```python
from build123d import *

# Parameters (mm, degrees)
SKETCH1_R           = 37.5
BOSS_EXTRUDE1_DEPTH = 65
CHAMFER1_SIZE       = 25
CHAMFER1_SIZE2      = 12.738136237
SKETCH3_R           = 21
CUT_EXTRUDE1_DEPTH  = 30
SKETCH4_R           = 35
CUT_EXTRUDE2_DEPTH  = 39
SKETCH5_R           = 24.761863763
BOSS_EXTRUDE3_DEPTH = 30
SKETCH6_R           = 21
CUT_EXTRUDE3_DEPTH  = 28
SKETCH7_R           = 20
CUT_EXTRUDE4_DEPTH  = 30


with BuildPart() as part:
    # Sketch1 → Boss-Extrude1 (new body)
    with BuildSketch(Plane(origin=(0, 0, 0), x_dir=(1, 0, 0), z_dir=(0, 1, 0))):
        with Locations(Location((0, 0, 0), (0, 0, 270))):
            Circle(SKETCH1_R)
    extrude(amount=BOSS_EXTRUDE1_DEPTH)

    # Chamfer1
    chamfer1_edges = [part.edges().sort_by_distance(p)[0] for p in [
        (0, 65, -37.5),
    ]]
    chamfer1_side = [part.faces().sort_by_distance(p)[0] for p in [
        (0, 32.5, -37.5),
    ]]
    chamfer(chamfer1_edges, length=CHAMFER1_SIZE, length2=CHAMFER1_SIZE2, reference=chamfer1_side[0])

    # Sketch3 → Cut-Extrude1 (cut)
    with BuildSketch(Plane(origin=(0, 65, 0), x_dir=(1, 0, 0), z_dir=(0, 1, 0))):
        with Locations(Location((0, 0, 0), (0, 0, 270))):
            Circle(SKETCH3_R)
    extrude(amount=-CUT_EXTRUDE1_DEPTH, mode=Mode.SUBTRACT)

    # Sketch4 → Cut-Extrude2 (cut)
    with BuildSketch(Plane.XZ):
        with Locations(Location((0, 0, 0), (0, 0, 270))):
            Circle(SKETCH4_R)
    extrude(amount=-CUT_EXTRUDE2_DEPTH, mode=Mode.SUBTRACT)

    # Sketch5 → Boss-Extrude3 (add)
    with BuildSketch(Plane(origin=(0, 65, 0), x_dir=(1, 0, 0), z_dir=(0, 1, 0))):
        with Locations(Location((0, 0, 0), (0, 0, 270))):
            Circle(SKETCH5_R)
    extrude(amount=BOSS_EXTRUDE3_DEPTH)

    # Sketch6 → Cut-Extrude3 (cut)
    with BuildSketch(Plane(origin=(0, 95, 0), x_dir=(1, 0, 0), z_dir=(0, 1, 0))):
        with Locations(Location((0, 0, 0), (0, 0, 270))):
            Circle(SKETCH6_R)
    extrude(amount=-CUT_EXTRUDE3_DEPTH, mode=Mode.SUBTRACT)

    # Sketch7 → Cut-Extrude4 (cut)
    with BuildSketch(Plane(origin=(0, 67, 0), x_dir=(1, 0, 0), z_dir=(0, 1, 0))):
        with Locations(Location((0, 0, 0), (0, 0, 270))):
            Circle(SKETCH7_R)
    extrude(amount=-CUT_EXTRUDE4_DEPTH, mode=Mode.SUBTRACT)


solid = part.part
```
Geometry check sheet. Reference: the model listing, model coordinates, mm. A direction names the side the tool comes from. Coordinates: 2 decimals unless noted, no trailing zeros. Loops run counter-clockwise (first coordinate to the right, second up) from the corner with the lowest first, then second, coordinate; pieces in that order, holes last. Notation, with made-up numbers: (63.25, 0.25) -> (68.25, 0.25) arc R25 cw to (68.25, 12.25) -> close; hole circle Ø6 at (88.25, 43). An arc over 180 degrees is marked (long way). Put each result on its own line as item: value.
1) Cross-section at A-A on x = 0. Record the boundary of the cut face in (y, z), plus the area to 3 significant figures.
Result set:
outline: (0, -37.5) -> (40, -37.5) -> (65, -24.76) -> (95, -24.76) -> (95, -21) -> (67, -21) -> (67, -20) -> (65, -20) -> (65, -21) -> (39, -21) -> (39, -35) -> (0, -35) -> close; (0, 35) -> (39, 35) -> (39, 21) -> (65, 21) -> (65, 20) -> (67, 20) -> (67, 21) -> (95, 21) -> (95, 24.76) -> (65, 24.76) -> (40, 37.5) -> (0, 37.5) -> close
area: 964 mm^2
2) Cross-section at B-B on z = 0. Record the boundary of the cut face in (x, y).
Result set:
outline: (-37.5, 0) -> (-35, 0) -> (-35, 39) -> (-21, 39) -> (-21, 65) -> (-20, 65) -> (-20, 67) -> (-21, 67) -> (-21, 95) -> (-24.76, 95) -> (-24.76, 65) -> (-37.5, 40) -> close; (20, 65) -> (21, 65) -> (21, 39) -> (35, 39) -> (35, 0) -> (37.5, 0) -> (37.5, 40) -> (24.76, 65) -> (24.76, 95) -> (21, 95) -> (21, 67) -> (20, 67) -> close
3) Thickness scan on line 1 (X direction, y = 10, z = 0); line 2 (X direction, y = 84.75, z = 0); line 3 (Z direction, x = -18, y = 32.5). Record the ranges inside material, lowest first.
Result set:
line 1: x = -37.5 to -35, 35 to 37.5
line 2: x = -24.76 to -21, 21 to 24.76
line 3: z = -32.9 to -30.02, 30.02 to 32.9
4) Tool access check on faces 1 (the cylindrical face through (-21, 19, 28)), 2 (the flat face through (17, 0, -31)), 3 (the flat face through (-8, 67, 19)). Record the directions out of +Z, -Z, +X, -X, +Y, -Y that give a thin tool (end or side, any length) a straight path to the whole face; none if there is none.
Result set:
face 1: -Y
face 2: +Z, -Z, +X, -X, -Y
face 3: +Y
5) Release check for a two-part mould opening along X. For faces 4 (the cylindrical face through (7.438, 79.79, 23.618)), 5 (the cylindrical face through (-19.524, 66.014, -4.336)), 6 (the flat face through (-18.2, 95, -11.1)) record: released by +X, released by -X, zero draft, split by the parting line, or undercut.
Result set:
face 4: split by the parting line
face 5: undercut
face 6: zero draft
6) Cross-section at C-C on y = 33. Record the boundary of the cut face in (x, z).
Result set:
outline: circle Ø75 at (0, 0); hole circle Ø70 at (0, 0)
7) Gauge pin test, flat ends, axial feed: pin 1 Ø2 at (x, y) = (28.5, 23.5) entering from -Z; pin 2 Ø4 at (x, y) = (-10.5, 51) entering from +Z; pin 3 Ø6 at (x, y) = (9, 64) entering from +Z. Record the tip position at first contact, or that the pin passes through.
Result set:
pin 1: stops at z = -25.5
pin 2: stops at z = 31.37
pin 3: stops at z = 25.52
